Autodesk Fusion 360 part; units mm, degrees
sketch "Sketch1" plane through (0, 0, 0) normal (0, 0, 1) x (1, 0, 0)
  line L0 (-52.5, 35) -> (52.5, 35)
  line L1 (52.5, 35) -> (52.5, -35)
  line L2 (52.5, -35) -> (-52.5, -35)
  line L3 (-52.5, -35) -> (-52.5, 35)
  line L4 (-55.5, 38) -> (55.5, 38)
  line L5 (55.5, 38) -> (55.5, -38)
  line L6 (55.5, -38) -> (-55.5, -38)
  line L7 (-55.5, -38) -> (-55.5, 38)
  dimension "d1" = 105
  dimension "d2" = 70
  dimension "d3" = 35
  dimension "d4" = 52.5
  dimension "d5" = 111
  dimension "d6" = 76
  dimension "d7" = 3
  dimension "d8" = 3
extrude "Extrude1" add sketch "Sketch1" along normal blind 3 contours L0 L1 L2 L3 makes body 1
extrude "Extrude2" add sketch "Sketch1" along normal blind 40 bodies 1
fillet "Fillet1" radius 4 4 edges at (55.5, -38, 20) (55.5, 38, 20) (-55.5, -38, 20) (-55.5, 38, 20) on bodies 1
fillet "Fillet2" radius 2.5 8 edges at (54.3284, -36.8284, 40) (55.5, 0, 40) (54.3284, 36.8284, 40) (0, 38, 40) (-54.3284, 36.8284, 40) (-55.5, 0, 40) (-54.3284, -36.8284, 40) (0, -38, 40) on bodies 1
sketch "Sketch3" plane through (0, -38, 0) normal (0, -1, 0) x (1, 0, 0)
  line L0 (51.5, 37.5) -> (-51.5, 37.5)
  line L1 (-51.5, 37.5) -> (-51.5, 0)
  line L2 (-51.5, 0) -> (51.5, 0)
  line L3 (51.5, 0) -> (51.5, 37.5)
  line L4 (-3.5, 11) -> (11.5, 11)
  line L5 (11.5, 11) -> (11.5, 4)
  line L6 (11.5, 4) -> (-3.5, 4)
  line L7 (-3.5, 4) -> (-3.5, 11)
  dimension "d17" = 7
  dimension "d19" = 40
  dimension "d22" = 11
  dimension "d23" = 15
extrude "Extrude3" cut sketch "Sketch3" against normal blind 10 contours L4 L5 L6 L7 bodies 1
sketch "Sketch5" plane through (0, 0, 40) normal (0, 0, 1) x (-1, 0, 0)
  line L0 (-52.5, 35) -> (52.5, 35)
  line L1 (52.5, 35) -> (52.5, -35)
  line L2 (52.5, -35) -> (-52.5, -35)
  line L3 (-52.5, -35) -> (-52.5, 35)
  arc A0 (-51.5, 35.5) -> (-53, 34) centre (-51.5, 34) ccw
  line L4 (-53, 34) -> (-53, -34)
  arc A1 (-53, -34) -> (-51.5, -35.5) centre (-51.5, -34) ccw
  line L5 (-51.5, -35.5) -> (51.5, -35.5)
  arc A2 (51.5, -35.5) -> (53, -34) centre (51.5, -34) ccw
  line L6 (53, -34) -> (53, 34)
  arc A3 (53, 34) -> (51.5, 35.5) centre (51.5, 34) ccw
  line L7 (51.5, 35.5) -> (-51.5, 35.5)
extrude "Extrude4" add sketch "Sketch5" against normal blind 2 separate body contours L0 L1 L2 L3 makes body 2
move_body "Move1" bodies 2 to x (1, 0, 0) y (0, 1, 0) z (0, 0, 1) at (0, 0, -3)
shell "Shell1" thickness 3 removed faces 2 at (17.5, -11.6667, 37) at (17.5, -11.6667, 35) on bodies 2
combine "Combine1" operation add target body 1 tool bodies 2
fillet "Fillet3" radius 2 4 edges at (-52.5, 35, 38.5) (-52.5, -35, 38.5) (52.5, -35, 38.5) (52.5, 35, 38.5) on bodies 1
Read the model definition and answer for the solid it produces. Units are mm, in the model's axes. A direction names the side the tool comes from. Give positions to 0.01 mm unless a question says otherwise; leave off trailing zeros. Write each loop counter-clockwise with the first axis right and the second up, starting at its lowest first coordinate (ties: lowest second). Pieces come first, ordered by that corner, then holes. Notation, with made-up numbers: M 20.5,12.5 L 75.5,12.5 A22 cw 75.5,48.5 Z; hole C 40.25,9 d8. An arc over 180 degrees is marked long. One line per item, written item: value. Start each with the question number.
(1) Find the intervals of material crossed by line 1 (X direction, y = 28, z = 27.5); line 2 (Y direction, x = 38.5, z = 17.5); line 3 (Z direction, x = 41.5, y = -33), in increasing order.
(2) Find section A-A (x = 9). Determine the outline of the cut face in (y, z), plus the area to 3 significant figures.
(3) A tool of negligible diameter and unlimited length cuts with its end or side. For faces 1 (the flat face through (52.5, 0, 19)), 2 (the flat face through (4, -37, 4)), 3 (the flat face through (-1, 35, 38)), from which of +Z, -Z, +X, -X, +Y, -Y can it reach the whole face along a straight path? Write none if from no direction.
(4) Flat-ended cylindrical pins translate along their axes: pin 1 Ø1.5 at (y, z) = (16, 38.5) entering from -X; pin 2 Ø3.5 at (y, z) = (-37, 6) entering from -X; pin 3 Ø1.5 at (y, z) = (-4.5, 39) entering from +X. Find the tip coordinate at first contact, or state that the pin passes through.
(5) Determine the mould class of faces 4 (the cylindrical face through (-54.297, 36.859, 19.012)), 5 (the cylindrical face through (-0.721, -37.287, 39.248)), 6 (the flat face through (-3.5, -37, 7)) for opening direction X: pulls with the +X half, pulls with the -X half, needs draft (parallel to the pull), parting line crosses it, or undercut.
(6) Find section D-D (x = -36.5). Determine the outline of the cut face in (y, z), plus the area to 3 significant figures.
(7) Find section B-B (z = 23.5). Determine the outline of the cut face in (x, y).
(8) Find section C-C (y = -25). Determine the outline of the cut face in (x, z).
Results below:
1. line 1: x = -55.5 to -52.5, 52.5 to 55.5
1. line 2: y = -38 to -35, 35 to 38
1. line 3: z = 0 to 3, 35 to 37
2. outline: M -38,0 L 38,0 L 38,37.5 A2.5 ccw 35.5,40 L 35,40 L 35,37 L 32,37 L 32,35 L 35,35 L 35,3 L -35,3 L -35,4 L -38,4 Z; M -38,11 L -35,11 L -35,35 L -32,35 L -32,37 L -35,37 L -35,40 L -35.5,40 A2.5 ccw -38,37.5 Z
2. area: 438 mm^2
3. face 1: none
3. face 2: -Y
3. face 3: +Z
4. pin 1: stops at x = -55.49
4. pin 2: stops at x = -55.3
4. pin 3: stops at x = 55.38
5. face 4: pulls with the -X half
5. face 5: needs draft
5. face 6: undercut
6. outline: M -38,0 L 38,0 L 38,37.5 A2.5 ccw 35.5,40 L 35,40 L 35,37 L 32,37 L 32,35 L 35,35 L 35,3 L -35,3 L -35,35 L -32,35 L -32,37 L -35,37 L -35,40 L -35.5,40 A2.5 ccw -38,37.5 Z
6. area: 459 mm^2
7. outline: M -55.5,-34 A4 ccw -51.5,-38 L 51.5,-38 A4 ccw 55.5,-34 L 55.5,34 A4 ccw 51.5,38 L -51.5,38 A4 ccw -55.5,34 Z; hole M -52.5,-35 L 52.5,-35 L 52.5,35 L -52.5,35 Z
8. outline: M -55.5,0 L 55.5,0 L 55.5,37.5 A2.5 ccw 53,40 L 52.5,40 L 52.5,37 L 49.5,37 L 49.5,35 L 52.5,35 L 52.5,3 L -52.5,3 L -52.5,35 L -49.5,35 L -49.5,37 L -52.5,37 L -52.5,40 L -53,40 A2.5 ccw -55.5,37.5 Z
